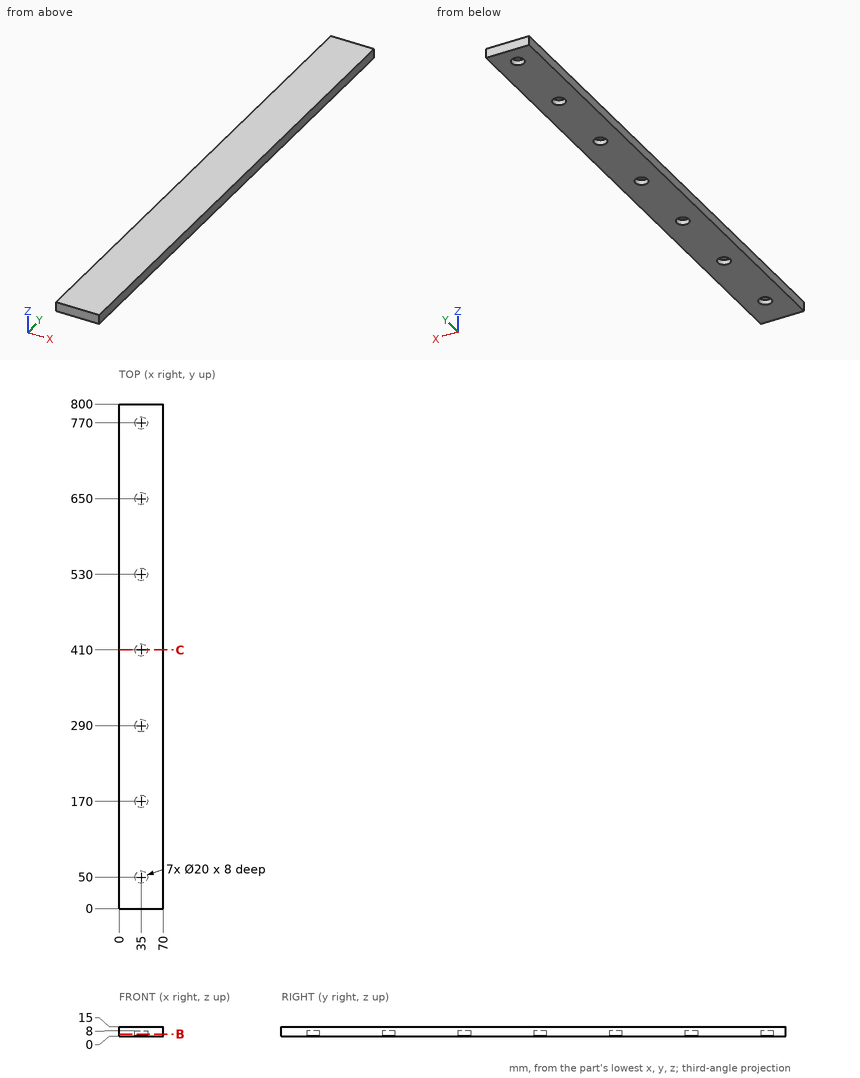
Design review of the part shown in the three views and the two pictorial views. Dimensions are in mm from the part's minimum x, y and z. Give positions to 0.01 mm unless a question says otherwise; leave off trailing zeros. Loops run counter-clockwise (first coordinate to the right, second up) from the corner with the lowest first, then second, coordinate; pieces in that order, holes last. Notation, with made-up numbers: (10.25, -30.75) -> (15.25, -30.75) arc R15 cw to (15.25, -12.75) -> close; hole circle Ø9 at (-32.5, -22). An arc over 180 degrees is marked (long way). One line per item, written item: value.
Q1. We need section C-C on y = 410. Give the boundary of the cut face in (x, z), and give its area (3 significant figures).
Numbers:
outline: (0, 0) -> (25, 0) -> (25, 8) -> (45, 8) -> (45, 0) -> (70, 0) -> (70, 15) -> (0, 15) -> close
area: 890 mm^2
Q2. For pin 1 Ø5 at (y, z) = (190.5, 3.5) entering from -X; pin 2 Ø18 at (x, y) = (35, 290) entering from -Z, all flat-tipped, find the tip position at first contact; note any pin that passes through.
Numbers:
pin 1: stops at x = 0
pin 2: stops at z = 8
Q3. For L1, parallel to X at y = 530, z = 6.5; L2, parallel to X at y = 766, z = 3.25, list the stretches that pass through material, from the lowest coordinate up.
Numbers:
L1: x = 0 to 25, 45 to 70
L2: x = 0 to 25.83, 44.17 to 70
Q4. We need section B-B on z = 3. Give the boundary of the cut face in (x, y), and give its area (3 significant figures).
Numbers:
outline: (0, 0) -> (70, 0) -> (70, 800) -> (0, 800) -> close; hole circle Ø20 at (35, 50); hole circle Ø20 at (35, 170); hole circle Ø20 at (35, 290); hole circle Ø20 at (35, 410); hole circle Ø20 at (35, 530); hole circle Ø20 at (35, 650); hole circle Ø20 at (35, 770)
area: 53,800 mm^2
